Geometry check sheet. Reference: drawing and pictorial views, mm from the part's lowest x, y, z. Give positions to 0.01 mm unless a question says otherwise; leave off trailing zeros. Write each loop counter-clockwise with the first axis right and the second up, starting at its lowest first coordinate (ties: lowest second). Pieces come first, ordered by that corner, then holes. Notation, with made-up numbers: M 86.5,14.25 L 95.5,14.25 A18 ccw 95.5,48.25 Z; hole C 72,-32 d7. An arc over 180 degrees is marked long. One line per item, written item: value. Start each with the question number.
1. Gauge pin test, flat ends, axial feed: pin 1 (5 mm diameter, centred on x = 47.5, z = 4, fed in from +Y); pin 2 (6 mm diameter, centred on x = 8, z = 5.5, fed in from +Y); pin 3 (4 mm diameter, centred on x = 7.5, z = 5.5, fed in from +Y) (1 decimal). Record the tip position at first contact, or that the pin passes through.
2. Release check for a two-part mould opening along Y. For the marked faces 1, 2 and 3 record: pulls with the +Y half, pulls with the -Y half, needs draft (parallel to the pull), parting line crosses it, or undercut.
3. Cross-section at A-A on z = 1.75. Record the cut outline in (x, y), then the cut area to 3 significant figures.
4. Scan lines: line 1 (Y direction, x = 26, z = 14); line 2 (Y direction, x = 33.5, z = 10) (1 decimal); line 3 (X direction, y = 22, z = 6.25). Record each from-to range of solid material in increasing order.
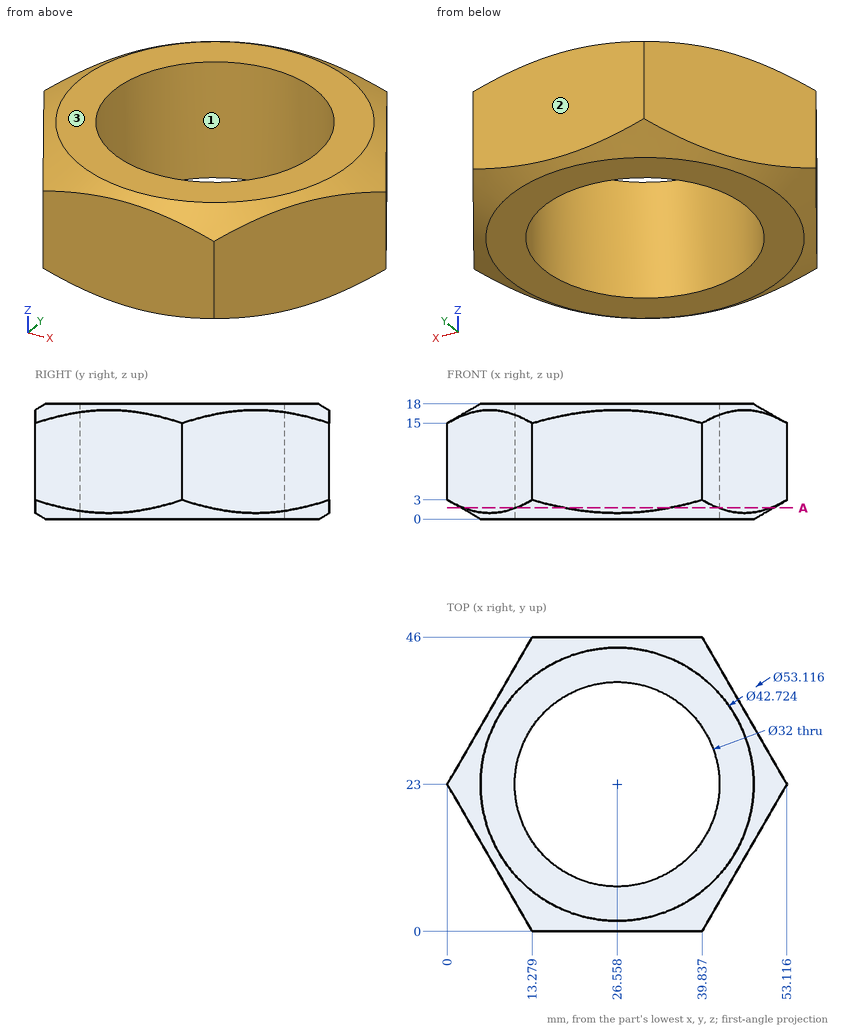
Report:
1. pin 1: stops at y = 37.06
1. pin 2: stops at y = 42.05
1. pin 3: stops at y = 39.5
2. face 1: undercut
2. face 2: pulls with the +Y half
2. face 3: needs draft
3. outline: M 2.58,18.54 L 10.7,4.46 A24.39 ccw 18.43,0 L 34.68,0 A24.39 ccw 42.41,4.46 L 50.54,18.54 A24.39 ccw 50.54,27.46 L 42.41,41.54 A24.39 ccw 34.68,46 L 18.43,46 A24.39 ccw 10.7,41.54 L 2.58,27.46 A24.39 ccw Z; hole C 26.56,23 d32
3. area: 974 mm^2
4. line 1: y = 0 to 7.01, 38.99 to 46
4. line 2: y = 0 to 8.6, 37.4 to 46
4. line 3: x = 0.58 to 10.59, 42.53 to 52.54
